```python
from build123d import *

# Parameters (mm, degrees)
F1_DEPTH = 76.2
F2_R     = 6.35
F3_DEPTH = 76.201
F4_R     = 6.35
F5_DEPTH = 76.201


with BuildPart() as f1:
    # F0 (on Right) → F1 (new body)
    with BuildSketch(Plane.YZ):
        Polygon((0, 76.2), (0, 0), (76.2, 0), (76.2, 6.35), (6.35, 6.35), (6.35, 76.2), align=None)
    extrude(amount=F1_DEPTH)

    # F2 (on Front) → F3 (cut, through all)
    with BuildSketch(Plane.XZ):
        with Locations((38.1, 57.15)):
            Circle(F2_R)
        with Locations((38.1, 38.1)):
            Circle(F2_R)
    extrude(amount=-F3_DEPTH, mode=Mode.SUBTRACT)

    # F4 (on Top) → F5 (cut, through all)
    with BuildSketch(Plane.XY):
        with Locations((38.1, 38.1)):
            Circle(F4_R)
        with Locations((38.1, 57.15)):
            Circle(F4_R)
    extrude(amount=F5_DEPTH, mode=Mode.SUBTRACT)


solid = f1.part
```
Check sheet for the modelled part. Datum: model origin and axes. Units: mm. A direction names the side the tool comes from. Coordinates: 2 decimals unless noted, no trailing zeros. Order: outer loops, then holes, each group sorted by start corner. A loop starts at its lowest first (then second) coordinate and runs counter-clockwise, first axis right, second up. Notation, with made-up numbers: (34.25, 13.25) -> (75.25, 13.25) arc R34 cw to (75.25, 51.25) -> close; hole circle Ø8 at (39, 28). An arc over 180 degrees is marked (long way). Write item = value, one per line. Start each with the question number.
1) Cross-section at A-A (z = 38.1). Enter the section's corners in (x, y), then the cut area to 3 significant figures.
2) Mould release check, pull along X, two halves, no side actions. Record for faces 3 (the cylindrical face through (33.06, 3.13, 53.29)), 4 (the flat face through (76.2, 4, 21)), 5 (the flat face through (38, 3, 76.2)), 6 (the cylindrical face through (33.06, 34.24, 3.13)): +X half, -X half, draft (parallel to the pull), parting line (faces both ways), or undercut.
3) Material ranges on L1, parallel to Y at x = 38, z = 4; L2, parallel to X at y = 38.1, z = 1.75, recorded low to high.
4) Go/stop test with flat-tipped pins: P1, Ø16.5, axis at x = 38.1, y = 57.15, coming from the +Z side; P2, Ø1, axis at x = 64.5, z = 41, coming from the -Y side; P3, Ø10, axis at y = 15, z = 59.5, coming from the -X side; P4, Ø16.5, axis at x = 38.1, z = 38.1, coming from the +Y side. Record where each tip stops, or that it passes through.
5) Access from +Z, -Z, +X, -X, +Y, -Y to the whole of each face (thin tool, end or side, straight path). Record for faces 1 (the flat face through (38, 6.35, 49)), 2 (the flat face through (38, 76.2, 3)).
6) Cross-section at D-D (x = 62). Enter the section's corners in (y, z), then the cut area to 3 significant figures.
7) Cross-section at B-B (x = 38.1). Enter the section's corners in (y, z), then the cut area to 3 significant figures.
Ans:
q1.outline = (0, 0) -> (31.75, 0) -> (31.75, 6.35) -> (0, 6.35) -> close; (44.45, 0) -> (76.2, 0) -> (76.2, 6.35) -> (44.45, 6.35) -> close
q1.area = 403 mm²
q2.face_3 = undercut
q2.face_4 = +X half
q2.face_5 = draft
q2.face_6 = undercut
q3.L1 = 0 to 31.75, 44.45 to 50.8, 63.5 to 76.2
q3.L2 = 0 to 31.75, 44.45 to 76.2
q4.P1 = 6.35
q4.P2 = 0
q4.P3 = through
q4.P4 = 6.35
q5.face_1 = +Z, +X, -X, +Y
q5.face_2 = +Z, -Z, +X, -X, +Y
q6.outline = (0, 0) -> (76.2, 0) -> (76.2, 6.35) -> (6.35, 6.35) -> (6.35, 76.2) -> (0, 76.2) -> close
q6.area = 927 mm²
q7.outline = (0, 0) -> (31.75, 0) -> (31.75, 6.35) -> (6.35, 6.35) -> (6.35, 31.75) -> (0, 31.75) -> close; (0, 44.45) -> (6.35, 44.45) -> (6.35, 50.8) -> (0, 50.8) -> close; (0, 63.5) -> (6.35, 63.5) -> (6.35, 76.2) -> (0, 76.2) -> close; (44.45, 0) -> (50.8, 0) -> (50.8, 6.35) -> (44.45, 6.35) -> close; (63.5, 0) -> (76.2, 0) -> (76.2, 6.35) -> (63.5, 6.35) -> close
q7.area = 605 mm²
